Autodesk Fusion 360 part; units mm, degrees
sketch "スケッチ1" plane through (0, 0, 0) normal (0, 0, 1) x (1, 0, 0)
  line L0 (0, 25) -> (50, 25)
  line L1 (50, -25) -> (0, -25)
  line L2 (0, -25) -> (0, 25)
  line L3 (50, 25) -> (50, 50)
  line L4 (50, 50) -> (100, 0)
  line L5 (100, 0) -> (50, -50)
  line L6 (50, -50) -> (50, -25)
  line L7 (0, 0) -> (100, 0) construction
  dimension "d2" = 100
  dimension "d3" = 50
  dimension "d4" = 50
  dimension "d5" = 100
extrude "押し出し1" add sketch "スケッチ1" along normal blind 5
Could you check a few things on this model? Use its own coordinates, in mm. A direction names the side the tool comes from. Round coordinates to 2 decimals unless told otherwise and drop trailing zeros. Loops run counter-clockwise (first coordinate to the right, second up) from the corner with the lowest first, then second, coordinate; pieces in that order, holes last. Notation, with made-up numbers: (50, -25) - (63, -25) arc R27 ccw to (63, 8) - close; hole circle Ø11 at (79.5, 43.25). An arc over 180 degrees is marked (long way). Answer as CSV lines item,"result".
1. I want a section at A-A on z = 2.55. List the corners of the cut face in (x, y) for me.
Filled in:
outline,"(0, -25) - (50, -25) - (50, -50) - (100, 0) - (50, 50) - (50, 25) - (0, 25) - close"
2. On a 3-axis mill with a long thin cutter (end or side, diameter ignored), from which of +Z, -Z, +X, -X, +Y, -Y can I reach the whole of each face in a straight line? I mean faces 1 (the face through (25, 25, 2)), 2 (the face through (25, -25, 2)), 3 (the face through (49, 1, 0)). Say none if no direction works.
Filled in:
face 1,"+Z, -Z, -X, +Y"
face 2,"+Z, -Z, -X, -Y"
face 3,"-Z, +X, -X, +Y, -Y"
3. Please list where these lines run through material, in increasing order: line 1 along Y through (x, z) = (7, 4.35); line 2 along Y through (x, z) = (50.5, 2.9); line 3 along X through (y, z) = (-6, 1.5). Write a range as [from, to].
Filled in:
line 1,"y = [-25, 25]"
line 2,"y = [-49.5, 49.5]"
line 3,"x = [0, 94]"
4. I want a section at C-C on y = 40. List the corners of the cut face in (x, z) for me, then the cut area to 3 significant figures.
Filled in:
outline,"(50, 0) - (60, 0) - (60, 5) - (50, 5) - close"
area,"50.0 mm^2"
5. For pin 1 Ø1.5 at (x, z) = (32.5, 3) entering from +Y; pin 2 Ø3 at (y, z) = (-30, 4) entering from +X; pin 3 Ø2.5 at (x, z) = (15.5, 3) entering from -Y, each with a flat end and sliding along its axis, tell me the tip position at first contact or that it passes through.
Filled in:
pin 1,"stops at y = 25"
pin 2,"stops at x = 71.5"
pin 3,"stops at y = -25"
6. I want a section at B-B on x = 41.5. List the corners of the cut face in (y, z) for me.
Filled in:
outline,"(-25, 0) - (25, 0) - (25, 5) - (-25, 5) - close"
